from build123d import *

# Parameters (mm, degrees)
SKETCH1_R           = 2
BOSS_EXTRUDE1_DEPTH = 5.2
SKETCH3_R           = 2
BOSS_EXTRUDE2_DEPTH = 0.15
BOSS_EXTRUDE2_TAPER = 45
SKETCH4_R           = 1.85
BOSS_EXTRUDE3_DEPTH = 0.5
SKETCH5_R           = 1.85
BOSS_EXTRUDE4_DEPTH = 0.15
BOSS_EXTRUDE4_DRAFT = -45
SKETCH6_R           = 2
BOSS_EXTRUDE5_DEPTH = 1.8
SKETCH7_R           = 2
BOSS_EXTRUDE6_DEPTH = 0.2
BOSS_EXTRUDE6_TAPER = 45
SKETCH11_R          = 1
CUT_EXTRUDE1_DEPTH  = 0.25
CUT_EXTRUDE1_DRAFT  = -45
SKETCH12_R          = 0.75
CUT_EXTRUDE2_DEPTH  = 4


with BuildPart() as part:
    # Sketch1 → Boss-Extrude1 (new body)
    with BuildSketch(Plane(origin=(0, 0, 0), x_dir=(1, 0, 0), z_dir=(0, 1, 0))):
        with Locations(Location((0, 0, 0), (0, 0, 270))):
            Circle(SKETCH1_R)
    extrude(amount=BOSS_EXTRUDE1_DEPTH)

    # Sketch3 → Boss-Extrude2 (add)
    with BuildSketch(Plane(origin=(0, 5.2, 0), x_dir=(1, 0, 0), z_dir=(0, 1, 0))):
        with Locations(Location((0, 0, 0), (0, 0, 270))):
            Circle(SKETCH3_R)
    extrude(amount=BOSS_EXTRUDE2_DEPTH, taper=BOSS_EXTRUDE2_TAPER)

    # Sketch4 → Boss-Extrude3 (add)
    with BuildSketch(Plane(origin=(0, 5.35, 0), x_dir=(1, 0, 0), z_dir=(0, 1, 0))):
        with Locations(Location((0, 0, 0), (0, 0, 270))):
            Circle(SKETCH4_R)
    extrude(amount=BOSS_EXTRUDE3_DEPTH)


with BuildPart() as boss_extrude4_tool:
    # Sketch5 → Boss-Extrude4 (with draft: the straight prism first)
    with BuildSketch(Plane(origin=(0, 5.85, 0), x_dir=(1, 0, 0), z_dir=(0, 1, 0))):
        with Locations(Location((0, 0, 0), (0, 0, 270))):
            Circle(SKETCH5_R)
    extrude(amount=BOSS_EXTRUDE4_DEPTH)
    # Boss-Extrude4: the draft: its side faces are tilted about the plane it starts from
    boss_extrude4_sides = [boss_extrude4_tool.faces().sort_by_distance(p)[0] for p in [
        (0, 5.925, -1.85),
    ]]
    draft(boss_extrude4_sides, Plane(origin=(0, 5.85, 0), x_dir=(1, 0, 0), z_dir=(0, 1, 0)), BOSS_EXTRUDE4_DRAFT)


with BuildPart() as part_1:
    add(part.part)

    # Boss-Extrude4: add boss_extrude4_tool
    add(boss_extrude4_tool.part)

    # Sketch6 → Boss-Extrude5 (add)
    with BuildSketch(Plane(origin=(0, 6, 0), x_dir=(1, 0, 0), z_dir=(0, 1, 0))):
        with Locations(Location((0, 0, 0), (0, 0, 270))):
            Circle(SKETCH6_R)
    extrude(amount=BOSS_EXTRUDE5_DEPTH)

    # Sketch7 → Boss-Extrude6 (add)
    with BuildSketch(Plane(origin=(0, 7.8, 0), x_dir=(1, 0, 0), z_dir=(0, 1, 0))):
        with Locations(Location((0, 0, 0), (0, 0, 270))):
            Circle(SKETCH7_R)
    extrude(amount=BOSS_EXTRUDE6_DEPTH, taper=BOSS_EXTRUDE6_TAPER)


with BuildPart() as cut_extrude1_tool:
    # Sketch11 → Cut-Extrude1 (with draft: the straight prism first)
    with BuildSketch(Plane(origin=(0, 8, 0), x_dir=(1, 0, 0), z_dir=(0, 1, 0))):
        Circle(SKETCH11_R)
    extrude(amount=-CUT_EXTRUDE1_DEPTH)
    # Cut-Extrude1: the draft: its side faces are tilted about the plane it starts from
    cut_extrude1_sides = [cut_extrude1_tool.faces().sort_by_distance(p)[0] for p in [
        (-1, 7.875, 0),
    ]]
    draft(cut_extrude1_sides, Plane(origin=(0, 8, 0), x_dir=(1, 0, 0), z_dir=(0, 1, 0)), CUT_EXTRUDE1_DRAFT)


with BuildPart() as part_2:
    add(part_1.part)

    # Cut-Extrude1: cut by cut_extrude1_tool
    add(cut_extrude1_tool.part, mode=Mode.SUBTRACT)

    # Sketch12 → Cut-Extrude2 (cut)
    with BuildSketch(Plane(origin=(0, 7.75, 0), x_dir=(1, 0, 0), z_dir=(0, 1, 0))):
        with Locations(Location((0, 0, 0), (0, 0, 270))):
            Circle(SKETCH12_R)
    extrude(amount=-CUT_EXTRUDE2_DEPTH, mode=Mode.SUBTRACT)


solid = part_2.part
Verification items for the finished model (mm, model axes). Give positions to 0.01 mm unless a question says otherwise; leave off trailing zeros. Loops run counter-clockwise (first coordinate to the right, second up) from the corner with the lowest first, then second, coordinate; pieces in that order, holes last.
1) Depth check by flat-ended pin: pin 1 Ø1.2 at (x, z) = (0, 0) entering from +Y; pin 2 Ø1 at (x, y) = (1, 1.5) entering from +Z; pin 3 Ø1.5 at (y, z) = (5.5, -1.5) entering from -X. Enter the tip coordinate at first touch or a pass-through.
2) Sectioned sample at C-C, the plane y = 1. Enter the section's corners in (x, z), then the cut area to 3 significant figures.
3) Sectioned sample at B-B, the plane z = 0. Enter the section's corners in (x, y), then the cut area to 3 significant figures.
4) Sectioned sample at A-A, the plane y = 4.75. Enter the section's corners in (x, z), then the cut area to 3 significant figures.
5) Draft check along Y on faces 1 (the flat face through (0, 3.75, 0)), 2 (the flat face through (0, 0, 0)), 3 (the cylindrical face through (0.225, 5.778, 0.715)), 4 (the cylindrical face through (-1.806, 5.596, -0.401)). Enter one of: pulls with the +Y half, pulls with the -Y half, needs draft (parallel to the pull), parting line crosses it, or undercut.
6) Thickness scan on line 1 along X through (y, z) = (6.15, 0); line 2 along Z through (x, y) = (0, 5.7). Record the ranges inside material, lowest first.
Answers:
1. pin 1: stops at y = 3.75
1. pin 2: stops at z = 1.94
1. pin 3: stops at x = -1.83
2. outline: circle Ø4 at (0, 0)
2. area: 12.6 mm2
3. outline: (-2, 0) - (2, 0) - (2, 5.2) - (1.85, 5.35) - (1.85, 5.85) - (2, 6) - (2, 7.8) - (1.8, 8) - (1, 8) - (0.75, 7.75) - (0.75, 3.75) - (-0.75, 3.75) - (-0.75, 7.75) - (-1, 8) - (-1.8, 8) - (-2, 7.8) - (-2, 6) - (-1.85, 5.85) - (-1.85, 5.35) - (-2, 5.2) - close
3. area: 25.3 mm2
4. outline: circle Ø4 at (0, 0); hole circle Ø1.5 at (0, 0)
4. area: 10.8 mm2
5. face 1: pulls with the +Y half
5. face 2: pulls with the -Y half
5. face 3: needs draft
5. face 4: undercut
6. line 1: x = -2 to -0.75, 0.75 to 2
6. line 2: z = -1.85 to -0.75, 0.75 to 1.85
